Design review of the part shown in the three views and the two pictorial views. Dimensions are in mm from the part's minimum x, y and z. Coordinates: 2 decimals unless noted, no trailing zeros. Write each loop counter-clockwise with the first axis right and the second up, starting at its lowest first coordinate (ties: lowest second). Pieces come first, ordered by that corner, then holes. Notation, with made-up numbers: (-38, 43) - (-34, 43) arc R35 cw to (-34, 75) - close; hole circle Ø1 at (14, 56.25). An arc over 180 degrees is marked (long way). Return JSON: item names as keys, results as strings. Group by question number.
(1) To check wall thickness, follow L1, parallel to X at y = 4, z = 24.5; L2, parallel to Z at x = 76.2, y = 6.25; L3, parallel to Z at x = 25, y = 8.25 (1 decimal). State the ranges of each line that lie inside material, in increasing order. Write a range as from..to.
(2) We need section A-A on x = 25.4. State the section outline as (y, z) points, then the cut area to 3 significant figures.
(3) For pin 1 Ø4 at (x, z) = (76.2, 23.06) entering from -Y, flat-tipped, find the tip position at first contact; note if it passes through.
(4) We need section B-B on z = 23.5. State the section outline as (x, y) points, then the cut area to 3 significant figures.
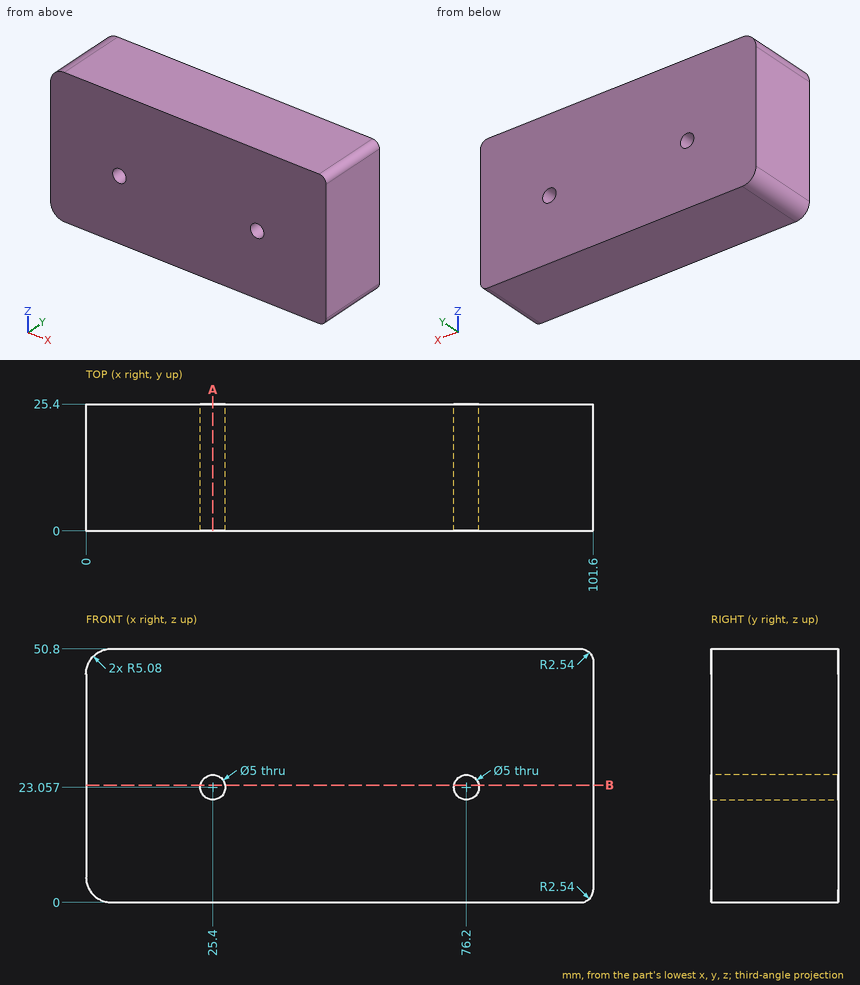
Ans:
{
 "1": {"L1": "0..23.36, 27.44..74.16, 78.24..101.6", "L2": "0..20.56, 25.56..50.8", "L3": "0..20.6, 25.5..50.8"},
 "2": {"outline": "(0, 0) - (25.4, 0) - (25.4, 20.56) - (0, 20.56) - close; (0, 25.56) - (25.4, 25.56) - (25.4, 50.8) - (0, 50.8) - close", "area": "1,160 mm²"},
 "3": {"pin 1": "through"},
 "4": {"outline": "(0, 0) - (22.94, 0) - (22.94, 25.4) - (0, 25.4) - close; (27.86, 0) - (73.74, 0) - (73.74, 25.4) - (27.86, 25.4) - close; (78.66, 0) - (101.6, 0) - (101.6, 25.4) - (78.66, 25.4) - close", "area": "2,330 mm²"}
}
